Check sheet for the drawn part. Datum: minimum x, y, z corner. Units: mm. A direction names the side the tool comes from. Give positions to 0.01 mm unless a question says otherwise; leave off trailing zeros. Write each loop counter-clockwise with the first axis right and the second up, starting at its lowest first coordinate (ties: lowest second). Pieces come first, ordered by that corner, then holes. Notation, with made-up numbers: (15.5, 46.5) - (47.5, 46.5) arc R26 ccw to (47.5, 60.5) - close; hole circle Ø6 at (61, -33.5). An arc over 180 degrees is marked (long way). Return JSON: item names as keys, results as strings. Group by question number.
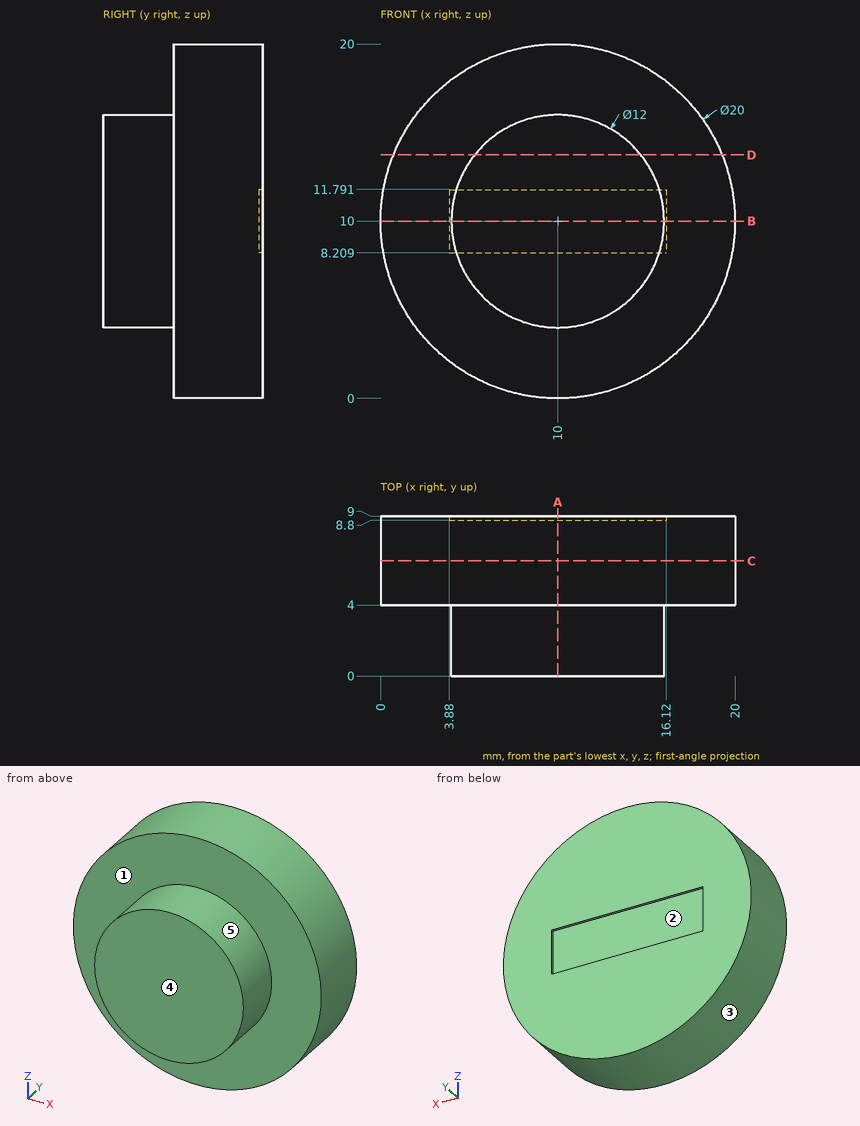
Item 1: Section check B-B on z = 10. Record the cut outline in (x, y), plus the area to 3 significant figures.
Item 2: Depth check by flat-ended pin: pin 1 (1 mm diameter, centred on y = 6, z = 5, fed in from +X); pin 2 (1 mm diameter, centred on y = 4, z = 12, fed in from -X); pin 3 (1.5 mm diameter, centred on x = 16.5, y = 8, fed in from -Z). Enter the tip coordinate at first touch or a pass-through.
Item 3: Access from +Z, -Z, +X, -X, +Y, -Y to the whole of each face (thin tool, end or side, straight path). Record for the marked faces 4 and 5.
Item 4: Section check D-D on z = 13.75. Record the cut outline in (x, y), plus the area to 3 significant figures.
Item 5: Mould release check, pull along Z, two halves, no side actions. Record for the marked faces 1, 2 and 3: +Z half, -Z half, draft (parallel to the pull), parting line (faces both ways), or undercut.
Item 6: Section check C-C on y = 6.5. Record the cut outline in (x, z), plus the area to 3 significant figures.
Item 7: Section check A-A on x = 10. Record the cut outline in (y, z).
Item 8: Material ranges on line 1 along Y through (x, z) = (19.25, 7.25); line 2 along Y through (x, z) = (12, 9.5); line 3 along X through (y, z) = (8.5, 13.25), recorded low to high. Write a range as from..to.
Reply:
{
 "1": {"outline": "(0, 4) - (4, 4) - (4, 0) - (16, 0) - (16, 4) - (20, 4) - (20, 9) - (16.12, 9) - (16.12, 8.8) - (3.88, 8.8) - (3.88, 9) - (0, 9) - close", "area": "146 mm²"},
 "2": {"pin 1": "x = 18.93", "pin 2": "x = 0.11", "pin 3": "z = 1.82"},
 "3": {"face 4": "+Z, -Z, +X, -X, -Y", "face 5": "-Y"},
 "4": {"outline": "(0.73, 4) - (5.32, 4) - (5.32, 0) - (14.68, 0) - (14.68, 4) - (19.27, 4) - (19.27, 9) - (0.73, 9) - close", "area": "130 mm²"},
 "5": {"face 1": "draft", "face 2": "undercut", "face 3": "parting line"},
 "6": {"outline": "circle Ø20 at (10, 10)", "area": "314 mm²"},
 "7": {"outline": "(0, 4) - (4, 4) - (4, 0) - (9, 0) - (9, 8.21) - (8.8, 8.21) - (8.8, 11.79) - (9, 11.79) - (9, 20) - (4, 20) - (4, 16) - (0, 16) - close"},
 "8": {"line 1": "4..9", "line 2": "0..8.8", "line 3": "0.54..19.46"}
}
